from build123d import *

# Parameters (mm, degrees)
SKETCH1_R           = 2.54
BOSS_EXTRUDE1_DEPTH = 12.7


with BuildPart() as part:
    # Sketch1 → Boss-Extrude1 (new body)
    with BuildSketch(Plane.XY):
        with BuildLine():
            Line((120.167455723, 128.44), (46.723424496, 128.44))
            add(Edge.make_bspline(
                [(46.723424496, 128.44), (44.179938737, 128.44), (44.179938737, 125.9)],
                knots=[1.570796327, 1.570796327, 1.570796327, 3.141592654, 3.141592654, 3.141592654], degree=2, weights=[1, 0.707106781, 1]))
            Line((44.179938737, 125.9), (44.179938737, 75.1))
            add(Edge.make_bspline(
                [(44.179938737, 75.1), (44.179938737, 72.56), (46.723424496, 72.56)],
                knots=[3.141592654, 3.141592654, 3.141592654, 4.71238898, 4.71238898, 4.71238898], degree=2, weights=[1, 0.707106781, 1]))
            Line((46.723424496, 72.56), (120.167455723, 72.56))
            ThreePointArc((120.167455723, 72.56), (121.963506947, 73.303948776), (122.707455723, 75.1))
            Line((122.707455723, 75.1), (122.707455723, 125.9))
            ThreePointArc((122.707455723, 125.9), (121.963506947, 127.696051224), (120.167455723, 128.44))
        make_face()
        with Locations((105.978138737, 79.8625)):
            Circle(SKETCH1_R, mode=Mode.SUBTRACT)
        with Locations((115.503138737, 79.8625)):
            Circle(SKETCH1_R, mode=Mode.SUBTRACT)
        with Locations((115.503138737, 121.1375)):
            Circle(SKETCH1_R, mode=Mode.SUBTRACT)
        with Locations((105.978138737, 121.1375)):
            Circle(SKETCH1_R, mode=Mode.SUBTRACT)
        with Locations((52.003138737, 121.1375)):
            Circle(SKETCH1_R, mode=Mode.SUBTRACT)
        with Locations((52.003138737, 79.8625)):
            Circle(SKETCH1_R, mode=Mode.SUBTRACT)
    extrude(amount=BOSS_EXTRUDE1_DEPTH)


solid = part.part
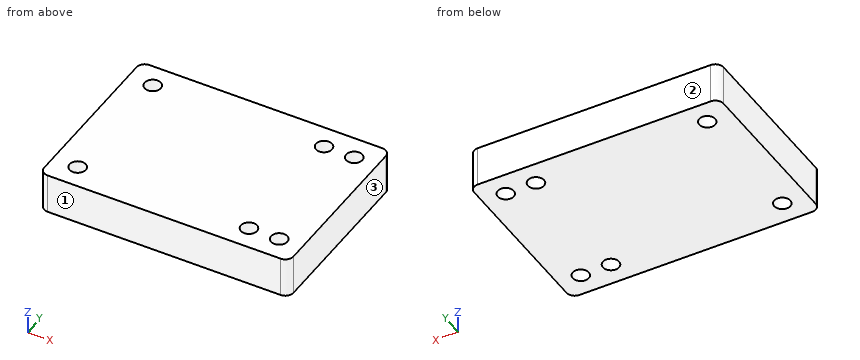
The listing builds one solid part. Answer for the finished solid, in the listing's coordinates (mm). Face numbers are marked on the shaded views. Coordinates: 2 decimals unless noted, no trailing zeros. Write each loop counter-clockwise with the first axis right and the second up, starting at its lowest first coordinate (ties: lowest second). Pieces come first, ordered by that corner, then holes. Notation, with made-up numbers: (40, 47) - (97, 47) arc R26 ccw to (97, 76) - close; hole circle Ø1 at (66, -39). An arc over 180 degrees is marked (long way). Return JSON: item names as keys, results as strings.
1. The part is cut by section C-C on z = 2.5. Count the separate pieces of the cut face and the enclosed holes in it, then the cut area to 3 significant figures.
Final values:
{"separate pieces": "1", "enclosed holes": "6", "area": "4,260 mm^2"}
2. The part is cut by section B-B on x = 116. Determine the outline of the cut face in (y, z).
Final values:
{"outline": "(72.56, 0) - (77.37, 0) - (77.37, 12.7) - (72.56, 12.7) - close; (82.35, 0) - (118.65, 0) - (118.65, 12.7) - (82.35, 12.7) - close; (123.63, 0) - (128.44, 0) - (128.44, 12.7) - (123.63, 12.7) - close"}
3. Consider line 1 along X through (y, z) = (119.5, 7); line 2 along Y through (x, z) = (53, 11.25); line 3 along X through (y, z) = (79.5, 7.25). Determine where each line is inside the solid, lowest interval first.
Final values:
{"line 1": "44.18 to 50.06, 53.94 to 104.04, 107.92 to 113.56, 117.44 to 122.71", "line 2": "72.56 to 77.53, 82.2 to 118.8, 123.47 to 128.44", "line 3": "44.18 to 49.49, 54.52 to 103.46, 108.49 to 112.99, 118.02 to 122.71"}
4. For a pull along Y with two mould halves and no side action, classify the marked faces 1, 2 and 3 as +Y half, -Y half, draft (parallel to the pull), parting line (faces both ways), or undercut.
Final values:
{"face 1": "-Y half", "face 2": "+Y half", "face 3": "draft"}
5. This flat-tipped pin is pushed along its axis until it touches: pin 1 Ø4.5 at (x, y) = (105.98, 121.14) entering from +Z. Where does it stop, or does it pass through?
Final values:
{"pin 1": "through"}
6. The part is cut by section A-A on y = 120. Determine the outline of the cut face in (x, z), then the cut area to 3 significant figures.
Final values:
{"outline": "(44.18, 0) - (49.73, 0) - (49.73, 12.7) - (44.18, 12.7) - close; (54.27, 0) - (103.71, 0) - (103.71, 12.7) - (54.27, 12.7) - close; (108.25, 0) - (113.23, 0) - (113.23, 12.7) - (108.25, 12.7) - close; (117.77, 0) - (122.71, 0) - (122.71, 12.7) - (117.77, 12.7) - close", "area": "824 mm^2"}
